Model file for the job. Use its own axes, mm. A direction names the side the tool comes from. Round coordinates to 2 decimals unless told otherwise and drop trailing zeros. Loops run counter-clockwise (first coordinate to the right, second up) from the corner with the lowest first, then second, coordinate; pieces in that order, holes last. Notation, with made-up numbers: M 87,11.5 L 102,11.5 A16 ccw 102,39.5 Z; hole C 44,48 d1. An arc over 180 degrees is marked long. Answer in a Markdown table with one row per item.
from build123d import *

# Parameters (mm, degrees)
SKETCH1_R           = 6
BOSS_EXTRUDE1_DEPTH = 4


with BuildPart() as part:
    # Sketch1 → Boss-Extrude1 (new body)
    with BuildSketch(Plane(origin=(0, 0, 0), x_dir=(1, 0, 0), z_dir=(0, 1, 0))):
        with BuildLine():
            Line((-2.5, -12.951833847), (-2.5, -31))
            Line((-2.5, -31), (2.5, -31))
            Line((2.5, -31), (2.5, -12.951833847))
            ThreePointArc((2.5, -12.951833847), (3.295532486, -9.043154047), (5.555555556, -5.756370599))
            ThreePointArc((5.555555556, -5.756370599), (0, 8), (-5.555555556, -5.756370599))
            ThreePointArc((-5.555555556, -5.756370599), (-3.295532486, -9.043154047), (-2.5, -12.951833847))
        make_face()
        Circle(SKETCH1_R, mode=Mode.SUBTRACT)
    extrude(amount=BOSS_EXTRUDE1_DEPTH)


solid = part.part
1. Tool access for faces 4 (the flat face through (-2.5, 2, 22)), 5 (the flat face through (0, 2, 31)), 6 (the flat face through (2.5, 2, 22)): list every direction of +Z, -Z, +X, -X, +Y, -Y with a clear straight run to the whole face (end or side of a thin tool).
Verdict:
| item | result |
|---|---|
| face 4 | +Z, -X, +Y, -Y |
| face 5 | +Z, +X, -X, +Y, -Y |
| face 6 | +Z, +X, +Y, -Y |
2. Saw through at C-C (z = 0). Write the cut outline in (x, y), and give its area (3 significant figures).
Verdict:
| item | result |
|---|---|
| outline | M -8,0 L -6,0 L -6,4 L -8,4 Z; M 6,0 L 8,0 L 8,4 L 6,4 Z |
| area | 16.0 mm² |
3. Saw through at B-B (y = 2.7). Write the cut outline in (x, z), and give its area (3 significant figures).
Verdict:
| item | result |
|---|---|
| outline | M -5.56,5.76 A8 ccw long 5.56,5.76 A10 cw 2.5,12.95 L 2.5,31 L -2.5,31 L -2.5,12.95 A10 cw Z; hole C 0,0 d12 |
| area | 211 mm² |
4. Mould opens along X. For faces 1 (the cylindrical face through (0, 2, -8)), 2 (the flat face through (0, 4, 11)), 3 (the cylindrical face through (-6, 2, 0)) say: +X half, -X half, draft (parallel to the pull), parting line (faces both ways), or undercut.
Verdict:
| item | result |
|---|---|
| face 1 | parting line |
| face 2 | draft |
| face 3 | undercut |
5. Saw through at A-A (x = 0). Write the cut outline in (y, z).
Verdict:
| item | result |
|---|---|
| outline | M 0,-8 L 4,-8 L 4,-6 L 0,-6 Z; M 0,6 L 4,6 L 4,31 L 0,31 Z |
6. Saw through at D-D (z = 21.5). Write the cut outline in (x, y), and give its area (3 significant figures).
Verdict:
| item | result |
|---|---|
| outline | M -2.5,0 L 2.5,0 L 2.5,4 L -2.5,4 Z |
| area | 20.0 mm² |
7. Pin check, flat tips, straight feed: pin 1 (2 mm diameter, centred on y = 3.5, z = 19, fed in from +X); pin 2 (1.5 mm diameter, centred on y = 2.5, z = 1.5, fed in from -X). Stop position of each tip, or through.
Verdict:
| item | result |
|---|---|
| pin 1 | stops at x = 2.5 |
| pin 2 | stops at x = -7.96 |
8. Wall check: probe 1 along Z at (x, y) = (0, 3.65); probe 2 along X at (y, z) = (2.45, 0); probe 3 along X at (y, z) = (2.5, -5.5). Give the ranges that are in metal, low to high.
Verdict:
| item | result |
|---|---|
| probe 1 | z = -8 to -6, 6 to 31 |
| probe 2 | x = -8 to -6, 6 to 8 |
| probe 3 | x = -5.81 to -2.4, 2.4 to 5.81 |
